For this review, take the finished solid that the model builds, in its own axes (mm). A direction names the side the tool comes from. Coordinates: 2 decimals unless noted, no trailing zeros. Write each loop counter-clockwise with the first axis right and the second up, starting at its lowest first coordinate (ties: lowest second). Pieces come first, ordered by that corner, then holes.
```python
from build123d import *

# Parameters (mm, degrees)
SKETCH1_W          = 5.715
SKETCH1_H          = 6.127
EXTRUDE1_DEPTH     = 12.83
SKETCH2_R          = 0.95
CUT_EXTRUDE1_DEPTH = 20.8
SKETCH4_W          = 0.8
SKETCH4_H          = 0.4
EXTRUDE2_DEPTH     = 3.1
EXTRUDE5_DEPTH     = 2.9


with BuildPart() as part:
    # Sketch1 → Extrude1 (new body)
    with BuildSketch(Plane(origin=(3.15, 0, 0), x_dir=(0, 0, -1), z_dir=(1, 0, 0))):
        with Locations((0.0425, 1.5635)):
            Rectangle(SKETCH1_W, SKETCH1_H)
    extrude(amount=-EXTRUDE1_DEPTH)

    # Sketch2 → Cut-Extrude1 (cut)
    with BuildSketch(Plane.XY.offset(2.815)):
        with Locations((0.085, -0.223)):
            Circle(SKETCH2_R)
        with Locations((-6.615, -0.223)):
            Circle(SKETCH2_R)
    extrude(amount=-CUT_EXTRUDE1_DEPTH, mode=Mode.SUBTRACT)

    # Sketch4 → Extrude2 (add)
    with BuildSketch(Plane.XZ.offset(1.5)):
        with Locations((-8.48, -0.0425)):
            Rectangle(SKETCH4_W, SKETCH4_H)
        with Locations((-3.265, -0.0425)):
            Rectangle(SKETCH4_W, SKETCH4_H)
        with Locations((1.95, -0.0425)):
            Rectangle(SKETCH4_W, SKETCH4_H)
    extrude(amount=EXTRUDE2_DEPTH)

    # Sketch7 → Extrude5 (add)
    with BuildSketch(Plane(origin=(0, 0, -1.45), x_dir=(-1, 0, 0), z_dir=(0, 0, -1))):
        with BuildLine():
            Line((7.755679036, 4.627), (6.400179952, 4.627))
            Line((6.400179952, 4.627), (6.400179952, 4.727))
            ThreePointArc((6.400179952, 4.727), (7.077929494, 5.259200233), (7.755679036, 4.727))
            Line((7.755679036, 4.727), (7.755679036, 4.627))
        make_face()
    extrude(amount=-EXTRUDE5_DEPTH)


solid = part.part
```
1) Consider section C-C (x = 0). Give the boundary of the cut face in (y, z) (3 decimals).
2) Clearance check with flat-ended pins moving along their axes: P1, Ø0.6, axis at x = 2, y = -3.5, coming from the -Z side; P2, Ø0.6, axis at x = -3, y = -3, coming from the +Z side. State where each tip first meets the part, or that it passes through.
3) For L1, parallel to X at y = -0.25, z = -1.2; L2, parallel to X at y = -3.25, z = -0.1 (3 decimals); L3, parallel to Y at x = -8.25, z = 0.6, list the stretches that pass through material, from the lowest coordinate up.
4) Consider section D-D (z = -0.75). Give the boundary of the cut face in (x, y) (3 decimals).
5) Consider section B-B (x = -3.5). Give the boundary of the cut face in (y, z) (1 decimal), then the cut area to 3 significant figures.
6) Consider section A-A (y = -4). Count the separate pieces of the cut face and the enclosed holes in it, then the cut area to 3 significant figures.
7) The part is to be moulded in two halves that separate along X. For faces 1 (the face through (2, -3, -0.243)), 2 (the face through (-9.68, 2, 0)), 3 (the face through (-0.615, 0.419, -0.002)), say which applies: pulls with the +X half, pulls with the -X half, needs draft (parallel to the pull), parting line crosses it, or undercut.
8) Tool access review of faces 4 (the face through (2, -3, 0.158)), 5 (the face through (-8.5, -3, -0.243)), 6 (the face through (3.15, 2, 0)): name each direction out of +Z, -Z, +X, -X, +Y, -Y from which nothing blocks a thin tool from reaching the whole face with its end or side.
Results:
1. outline: (-1.5, -2.9) - (-1.169, -2.9) - (-1.169, 2.815) - (-1.5, 2.815) - close; (0.723, -2.9) - (4.627, -2.9) - (4.627, 2.815) - (0.723, 2.815) - close
2. P1: stops at z = -0.24
2. P2: stops at z = 0.16
3. L1: x = -9.68 to -7.56, -5.67 to -0.86, 1.03 to 3.15
3. L2: x = -8.88 to -8.08, -3.665 to -2.865, 1.55 to 2.35
3. L3: y = -1.5 to 4.63
4. outline: (-9.68, -1.5) - (3.15, -1.5) - (3.15, 4.627) - (-6.4, 4.627) - (-6.4, 4.727) arc R0.698 ccw to (-7.756, 4.727) - (-7.756, 4.627) - (-9.68, 4.627) - close; hole circle Ø1.9 at (-6.615, -0.223); hole circle Ø1.9 at (0.085, -0.223)
5. outline: (-4.6, -0.2) - (-1.5, -0.2) - (-1.5, -2.9) - (4.6, -2.9) - (4.6, 2.8) - (-1.5, 2.8) - (-1.5, 0.2) - (-4.6, 0.2) - close
5. area: 36.3 mm2
6. separate pieces: 3
6. enclosed holes: 0
6. area: 0.960 mm2
7. face 1: needs draft
7. face 2: pulls with the -X half
7. face 3: undercut
8. face 4: +Z, +X, -X, -Y
8. face 5: -Z, +X, -X, -Y
8. face 6: +Z, -Z, +X, +Y, -Y
